```python
from build123d import *

# Parameters (mm, degrees)
SKETCH1_W           = 100
SKETCH1_H           = 22
BOSS_EXTRUDE1_DEPTH = 3
SKETCH2_R           = 1.7
CUT_EXTRUDE1_DEPTH  = 3
FILLET1_R           = 10
FILLET2_R           = 2


with BuildPart() as part:
    # Sketch1 → Boss-Extrude1 (new body)
    with BuildSketch(Plane(origin=(0, 12, 0), x_dir=(1, 0, 0), z_dir=(0, 1, 0))):
        with Locations((0, 39)):
            Rectangle(SKETCH1_W, SKETCH1_H)
    extrude(amount=BOSS_EXTRUDE1_DEPTH)

    # Sketch2 → Cut-Extrude1 (cut)
    with BuildSketch(Plane(origin=(0, 15, 0), x_dir=(1, 0, 0), z_dir=(0, 1, 0))):
        with Locations(Location((-21.5, 39, 0), (0, 0, 270))):
            Circle(SKETCH2_R)
        with Locations(Location((21.5, 39, 0), (0, 0, 270))):
            Circle(SKETCH2_R)
    extrude(amount=-CUT_EXTRUDE1_DEPTH, mode=Mode.SUBTRACT)

    # Fillet1
    fillet1_edges = [part.edges().sort_by_distance(p)[0] for p in [
        (-50, 13.5, -50),
        (50, 13.5, -50),
    ]]
    fillet(fillet1_edges, radius=FILLET1_R)

    # Fillet2
    fillet2_edges = [part.edges().sort_by_distance(p)[0] for p in [
        (50, 13.5, -28),
        (-50, 13.5, -28),
    ]]
    fillet(fillet2_edges, radius=FILLET2_R)


solid = part.part
```
Here's how the part is built. I have some questions about the finished solid (model axes, mm). Give positions to 0.01 mm unless a question says otherwise; leave off trailing zeros. Loops run counter-clockwise (first coordinate to the right, second up) from the corner with the lowest first, then second, coordinate; pieces in that order, holes last. Notation, with made-up numbers: M 19,27.25 L 58,27.25 A24 cw 58,48.25 Z; hole C 5,-30 d2. An arc over 180 degrees is marked long. Put each result on its own line as item: value. Start each with the question number.
(1) I want a section at C-C on y = 12.95. Please give me the cut outline in (x, z).
(2) I want a section at A-A on x = 21.5. Please give me the cut outline in (y, z).
(3) If we mould it in two halves opening along X, with no side actions, what happens to faces 1 (the cylindrical face through (22.65, 13.52, -40.25)), 2 (the cylindrical face through (-47.15, 13.52, -46.99)), 3 (the flat face through (50, 13, -35))? For each: +X half, -X half, draft (parallel to the pull), parting line (faces both ways), or undercut.
(4) I want a section at B-B on z = -39. Please give me the cut outline in (x, y).
(5) I need wall thicknesses on line 1 along X through (y, z) = (13.7, -39); line 2 along X through (y, z) = (14.4, -39.75); line 3 along X through (y, z) = (12.8, -41.75). Which ranges of each line are inside material? Lowest first, please. Write a range as [from, to].
Answer block:
1. outline: M -50,-40 A10 ccw -40,-50 L 40,-50 A10 ccw 50,-40 L 50,-30 A2 ccw 48,-28 L -48,-28 A2 ccw -50,-30 Z; hole C -21.5,-39 d3.4; hole C 21.5,-39 d3.4
2. outline: M 12,-50 L 15,-50 L 15,-40.7 L 12,-40.7 Z; M 12,-37.3 L 15,-37.3 L 15,-28 L 12,-28 Z
3. face 1: undercut
3. face 2: -X half
3. face 3: +X half
4. outline: M -50,12 L -23.2,12 L -23.2,15 L -50,15 Z; M -19.8,12 L 19.8,12 L 19.8,15 L -19.8,15 Z; M 23.2,12 L 50,12 L 50,15 L 23.2,15 Z
5. line 1: [-50, -23.2], [-19.8, 19.8], [23.2, 50]
5. line 2: [-50, -23.03], [-19.97, 19.97], [23.03, 50]
5. line 3: [-49.85, 49.85]
